Can you work these out from the model? Positions are in its coordinate system, mm. A direction names the side the tool comes from. Give positions to 0.01 mm unless a question says otherwise; leave off trailing zeros. Loops run counter-clockwise (first coordinate to the right, second up) from the corner with the lowest first, then second, coordinate; pieces in that order, holes last. Notation, with made-up numbers: (-10, 40) - (6, 40) arc R15 ccw to (6, 66) - close; hole circle Ø2 at (36.25, -6). An arc over 180 degrees is marked (long way). Answer as a JSON object with one key per item and string values.
```python
from build123d import *

# Parameters (mm, degrees)
SKETCH_1_W          = 10
SKETCH_1_H          = 10
SKETCH_1_W_2        = 6
SKETCH_1_H_2        = 6
EXTRUDE_1_DEPTH     = 150
SKETCH_2_R          = 1
CUT_EXTRUDE_1_DEPTH = 10
SKETCH_3_R          = 1
CUT_EXTRUDE_2_DEPTH = 10
SKETCH_4_R          = 1
CUT_EXTRUDE_3_DEPTH = 10
SKETCH_5_R          = 4
CUT_EXTRUDE_4_DEPTH = 150
SKETCH_6_R          = 1
CUT_EXTRUDE_5_DEPTH = 10


with BuildPart() as part:
    # 草图1 → 凸台-拉伸1 (new body)
    with BuildSketch(Plane(origin=(0, 0, 0), x_dir=(1, 0, 0), z_dir=(0, 1, 0))):
        with Locations((5, 5)):
            Rectangle(SKETCH_1_W, SKETCH_1_H)
        with Locations((5, 5)):
            Rectangle(SKETCH_1_W_2, SKETCH_1_H_2, mode=Mode.SUBTRACT)
    extrude(amount=EXTRUDE_1_DEPTH)

    # 草图2 → 切除-拉伸1 (cut)
    with BuildSketch(Plane.XY):
        with BuildLine():
            Line((4, 140), (4, 110))
            ThreePointArc((4, 110), (5, 111), (6, 110))
            Line((6, 110), (6, 140))
            ThreePointArc((6, 140), (5, 139), (4, 140))
        make_face()
        with Locations((5, 110)):
            Circle(SKETCH_2_R)
        with BuildLine():
            ThreePointArc((6, 140), (5, 141), (4, 140))
            Line((4, 140), (6, 140))
        make_face()
        with BuildLine():
            Line((6, 140), (4, 140))
            ThreePointArc((4, 140), (5, 139), (6, 140))
        make_face()
    extrude(amount=-CUT_EXTRUDE_1_DEPTH, mode=Mode.SUBTRACT)

    # 草图3 → 切除-拉伸2 (cut)
    with BuildSketch(Plane.XY):
        with Locations((5, 90)):
            Circle(SKETCH_3_R)
    extrude(amount=-CUT_EXTRUDE_2_DEPTH, mode=Mode.SUBTRACT)

    # 草图4 → 切除-拉伸3 (cut)
    with BuildSketch(Plane(origin=(0, 0, -10), x_dir=(-1, 0, 0), z_dir=(0, 0, -1))):
        with Locations((-5, 5)):
            Circle(SKETCH_4_R)
    extrude(amount=-CUT_EXTRUDE_3_DEPTH, mode=Mode.SUBTRACT)

    # 草图5 → 切除-拉伸4 (cut)
    with BuildSketch(Plane(origin=(0, 0, 0), x_dir=(1, 0, 0), z_dir=(0, 1, 0))):
        with BuildLine():
            Line((1, 9), (1, 5))
            ThreePointArc((1, 5), (2.171572875, 7.828427125), (5, 9))
            Line((5, 9), (1, 9))
        make_face()
        with Locations((5, 5)):
            Circle(SKETCH_5_R)
        with BuildLine():
            ThreePointArc((5, 1), (2.171572875, 2.171572875), (1, 5))
            Line((1, 5), (1, 1))
            Line((1, 1), (5, 1))
        make_face()
        with BuildLine():
            Line((9, 9), (5, 9))
            ThreePointArc((5, 9), (7.828427125, 7.828427125), (9, 5))
            Line((9, 5), (9, 9))
        make_face()
        with BuildLine():
            ThreePointArc((9, 5), (7.828427125, 2.171572875), (5, 1))
            Line((5, 1), (9, 1))
            Line((9, 1), (9, 5))
        make_face()
    extrude(amount=CUT_EXTRUDE_4_DEPTH, mode=Mode.SUBTRACT)

    # 草图6 → 切除-拉伸5 (cut)
    with BuildSketch(Plane(origin=(0, 0, -10), x_dir=(-1, 0, 0), z_dir=(0, 0, -1))):
        with Locations((-5, 50)):
            Circle(SKETCH_6_R)
    extrude(amount=-CUT_EXTRUDE_5_DEPTH, mode=Mode.SUBTRACT)


solid = part.part
```
1) Which directions (+Z, -Z, +X, -X, +Y, -Y) give clear straight access to the entire face, cutting with the end or side of a thin tool? Please do faces 1 (the flat face through (1, 74, -5)), 2 (the flat face through (0.5, 0, -5.1)).
Check sheet entries:
{"face 1": "+Y, -Y", "face 2": "+Z, -Z, +X, -X, -Y"}
2) If we mould it in two halves opening along Z, with no side actions, what happens to faces 3 (the flat face through (9, 74, -5)), 4 (the flat face through (5, 74, 0)), 5 (the flat face through (0.5, 150, -5.1))? For each: released by +Z, released by -Z, zero draft, split by the parting line, or undercut.
Check sheet entries:
{"face 3": "undercut", "face 4": "released by +Z", "face 5": "zero draft"}
3) Imagine slicing it at A-A on z = -5.25. Write out the boundary of the cut face in (x, y).
Check sheet entries:
{"outline": "(0, 0) - (1, 0) - (1, 150) - (0, 150) - close; (9, 0) - (10, 0) - (10, 150) - (9, 150) - close"}
4) Imagine slicing it at B-B on y = 24. Write out the boundary of the cut face in (x, z).
Check sheet entries:
{"outline": "(0, -10) - (10, -10) - (10, 0) - (0, 0) - close; hole (1, -9) - (9, -9) - (9, -1) - (1, -1) - close"}
5) I need wall thicknesses on L1, parallel to Y at x = 5, z = -9.25; L2, parallel to X at y = 72, z = -8; L3, parallel to Z at x = 5, y = 15. Which ranges of each line are inside material? Lowest first, please.
Check sheet entries:
{"L1": "0 to 4, 6 to 49, 51 to 89, 91 to 109, 141 to 150", "L2": "0 to 1, 9 to 10", "L3": "-10 to -9, -1 to 0"}
